```python
from build123d import *

# Parameters (mm, degrees)
SZKIC1_W                    = 77.4
SZKIC1_H                    = 77.4
DODANIE_WYCI_GNI_CIE1_DEPTH = 6
DODANIE_WYCI_GNI_CIE2_DEPTH = 30
ZAOKR_GLENIE1_R             = 10


with BuildPart() as part:
    # Szkic1 → Dodanie-wyciągnięcie1 (new body)
    with BuildSketch(Plane(origin=(0, 0, 0), x_dir=(1, 0, 0), z_dir=(0, 1, 0))):
        Rectangle(SZKIC1_W, SZKIC1_H)
    extrude(amount=-DODANIE_WYCI_GNI_CIE1_DEPTH)

    # Szkic2 → Dodanie-wyciągnięcie2 (add)
    with BuildSketch(Plane.XZ.offset(6)):
        with BuildLine():
            Line((-30, -35), (30, -35))
            ThreePointArc((30, -35), (33.535533906, -33.535533906), (35, -30))
            Line((35, -30), (35, 30))
            ThreePointArc((35, 30), (33.535533906, 33.535533906), (30, 35))
            Line((30, 35), (-30, 35))
            ThreePointArc((-30, 35), (-33.535533906, 33.535533906), (-35, 30))
            Line((-35, 30), (-35, -30))
            ThreePointArc((-35, -30), (-33.535533906, -33.535533906), (-30, -35))
        make_face()
        with BuildLine():
            Line((-33, -30), (-33, 30))
            ThreePointArc((-33, 30), (-32.121320344, 32.121320344), (-30, 33))
            Line((-30, 33), (30, 33))
            ThreePointArc((30, 33), (32.121320344, 32.121320344), (33, 30))
            Line((33, 30), (33, -30))
            ThreePointArc((33, -30), (32.121320344, -32.121320344), (30, -33))
            Line((30, -33), (-30, -33))
            ThreePointArc((-30, -33), (-32.121320344, -32.121320344), (-33, -30))
        make_face(mode=Mode.SUBTRACT)
    extrude(amount=DODANIE_WYCI_GNI_CIE2_DEPTH)

    # Zaokrąglenie1
    zaokr_glenie1_edges = [part.edges().sort_by_distance(p)[0] for p in [
        (38.7, -3, 38.7),
        (-38.7, -3, 38.7),
        (-38.7, -3, -38.7),
        (38.7, -3, -38.7),
    ]]
    fillet(zaokr_glenie1_edges, radius=ZAOKR_GLENIE1_R)


solid = part.part
```
Could you check a few things on this model? Use its own coordinates, in mm. A direction names the side the tool comes from. Round coordinates to 2 decimals unless told otherwise and drop trailing zeros. Order: outer loops, then holes, each group sorted by start corner. A loop starts at its lowest first (then second) coordinate and runs counter-clockwise, first axis right, second up. Notation, with made-up numbers: M 21,-8 L 54,-8 A23 ccw 54,22 Z; hole C -21,-17.75 d9. An arc over 180 degrees is marked long. One line per question, with ' | ' between items. Start each with the question number.
(1) Suppose I cut it at C-C on z = 18. List the corners of the cut face in (x, y) for me.
(2) Suppose I cut it at B-B on x = 25. List the corners of the cut face in (y, z) for me, then the cut area to 3 significant figures.
(3) Thinking about a two-plate mould opening in X: for faces 1 (the face through (-35, -21, 0)), 2 (the face through (35.69, -3.04, -35.85)), 3 (the face through (0, -6, 0)), 4 (the face through (32.1, -20.79, 32.14)), which applies, +X half, -X half, draft (parallel to the pull), parting line (faces both ways), or undercut?
(4) For faces 5 (the face through (0, -6, -37)), 6 (the face through (34, -21, 33)), 7 (the face through (0, -21, 35)), which set-ups out of +Z, -Z, +X, -X, +Y, -Y let a thin tool reach every point of the face, with its end or its side?
(5) For P1, Ø10, axis at x = 26.5, y = -20.5, coming from the -Z side; P2, Ø9, axis at x = 7, y = -25.5, coming from the +Z side; P3, Ø8, axis at x = 17.5, z = -1, coming from the -Y side, each with a flat end and sliding along its axis, tell me the tip position at first contact or that it passes through.
(6) Suppose I cut it at D-D on x = -34. List the corners of the cut face in (y, z) for me, then the cut area to 3 significant figures.
(7) Suppose I cut it at A-A on y = -9. List the corners of the cut face in (x, z) for me, then the cut area to 3 significant figures.
(8) Please list where these lines run through material, in increasing order: line 1 along Z through (x, y) = (1, -24.5); line 2 along Y through (x, z) = (24, 9.5).
Geometry results:
1) outline: M -38.7,-6 L -35,-6 L -35,-36 L -33,-36 L -33,-6 L 33,-6 L 33,-36 L 35,-36 L 35,-6 L 38.7,-6 L 38.7,0 L -38.7,0 Z
2) outline: M -36,-35 L -6,-35 L -6,-38.7 L 0,-38.7 L 0,38.7 L -6,38.7 L -6,35 L -36,35 L -36,33 L -6,33 L -6,-33 L -36,-33 Z | area: 584 mm²
3) face 1: -X half | face 2: +X half | face 3: undercut | face 4: undercut
4) face 5: -Y | face 6: +Z, +X, -Y | face 7: +Z, +X, -X, -Y
5) P1: z = -35 | P2: z = 35 | P3: y = -6
6) outline: M -36,-33 L -6,-33 L -6,-37.18 L 0,-37.18 L 0,37.18 L -6,37.18 L -6,33 L -36,33 Z | area: 2,430 mm²
7) outline: M -35,-30 A5 ccw -30,-35 L 30,-35 A5 ccw 35,-30 L 35,30 A5 ccw 30,35 L -30,35 A5 ccw -35,30 Z; hole M -33,-30 A3 ccw -30,-33 L 30,-33 A3 ccw 33,-30 L 33,30 A3 ccw 30,33 L -30,33 A3 ccw -33,30 Z | area: 530 mm²
8) line 1: -35 to -33, 33 to 35 | line 2: -6 to 0
